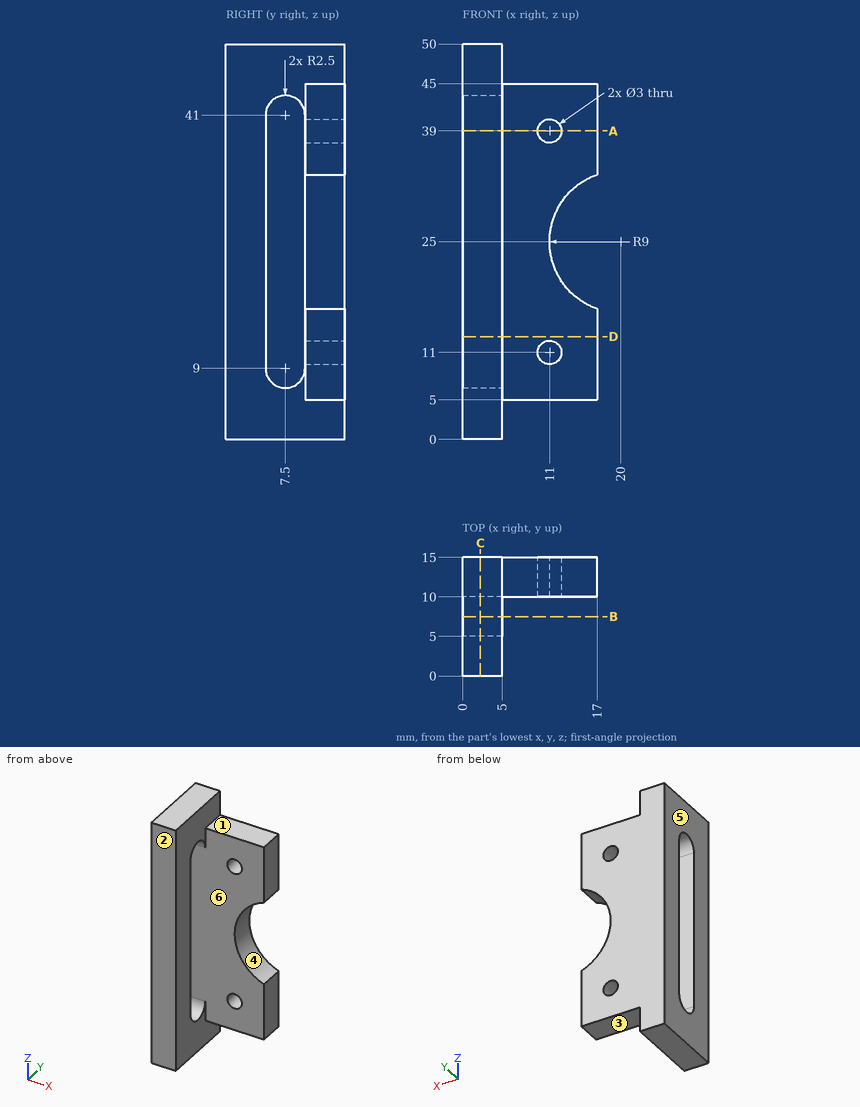
Verification items for this drawing (mm, ordinates from the low corner). A direction names the side the tool comes from. Round coordinates to 2 decimals unless told otherwise and drop trailing zeros. Loops run counter-clockwise (first coordinate to the right, second up) from the corner with the lowest first, then second, coordinate; pieces in that order, holes last. Notation, with made-up numbers: (-12, 79.5) -> (11, 79.5) arc R16 ccw to (11, 91.5) -> close; hole circle Ø2 at (56, -24.5). An arc over 180 degrees is marked (long way). Answer in a Markdown table with one row per item.
Q1. Release check for a two-part mould opening along Z. For the marked faces 3, 4, 5 and 6 record: released by +Z, released by -Z, zero draft, split by the parting line, or undercut.
Data:
| item | result |
|---|---|
| face 3 | released by -Z |
| face 4 | undercut |
| face 5 | zero draft |
| face 6 | undercut |
Q2. Set-up check for the marked faces 1 and 2: record each of +Z, -Z, +X, -X, +Y, -Y from which the full face is reachable in a straight line by a thin tool's end or side.
Data:
| item | result |
|---|---|
| face 1 | +Z, +X, +Y, -Y |
| face 2 | +Z, -Z, +X, -X, -Y |
Q3. Sectioned sample at B-B on y = 7.5. Enter the section's corners in (x, z), then the cut area to 3 significant figures.
Data:
| item | result |
|---|---|
| outline | (0, 0) -> (5, 0) -> (5, 6.5) -> (0, 6.5) -> close; (0, 43.5) -> (5, 43.5) -> (5, 50) -> (0, 50) -> close |
| area | 65.0 mm^2 |
Q4. Go/stop test with flat-tipped pins: P1, Ø1.5, axis at x = 8.5, y = 12.5, coming from the +Z side; P2, Ø5.5, axis at x = 10, y = 11.5, coming from the -Z side; P3, Ø5, axis at x = 11, z = 11, coming from the -Y side. Record where each tip stops, or that it passes through.
Data:
| item | result |
|---|---|
| P1 | stops at z = 45 |
| P2 | stops at z = 5 |
| P3 | stops at y = 10 |
Q5. Sectioned sample at C-C on x = 2.25. Enter the section's corners in (y, z).
Data:
| item | result |
|---|---|
| outline | (0, 0) -> (15, 0) -> (15, 50) -> (0, 50) -> close; hole (5, 9) arc R2.5 ccw to (10, 9) -> (10, 41) arc R2.5 ccw to (5, 41) -> close |
Q6. Sectioned sample at A-A on z = 39. Enter the section's corners in (x, y), then the cut area to 3 significant figures.
Data:
| item | result |
|---|---|
| outline | (0, 0) -> (5, 0) -> (5, 5) -> (0, 5) -> close; (0, 10) -> (9.5, 10) -> (9.5, 15) -> (0, 15) -> close; (12.5, 10) -> (17, 10) -> (17, 15) -> (12.5, 15) -> close |
| area | 95.0 mm^2 |
Q7. Thickness scan on L1, parallel to X at y = 13.35, z = 39; L2, parallel to Y at x = 1.5, z = 18.5; L3, parallel to X at y = 1.75, z = 8.5. Record the ranges inside material, lowest first.
Data:
| item | result |
|---|---|
| L1 | x = 0 to 9.5, 12.5 to 17 |
| L2 | y = 0 to 5, 10 to 15 |
| L3 | x = 0 to 5 |
Q8. Sectioned sample at D-D on z = 13. Enter the section's corners in (x, y), then the cut area to 3 significant figures.
Data:
| item | result |
|---|---|
| outline | (0, 0) -> (5, 0) -> (5, 5) -> (0, 5) -> close; (0, 10) -> (17, 10) -> (17, 15) -> (0, 15) -> close |
| area | 110 mm^2 |
